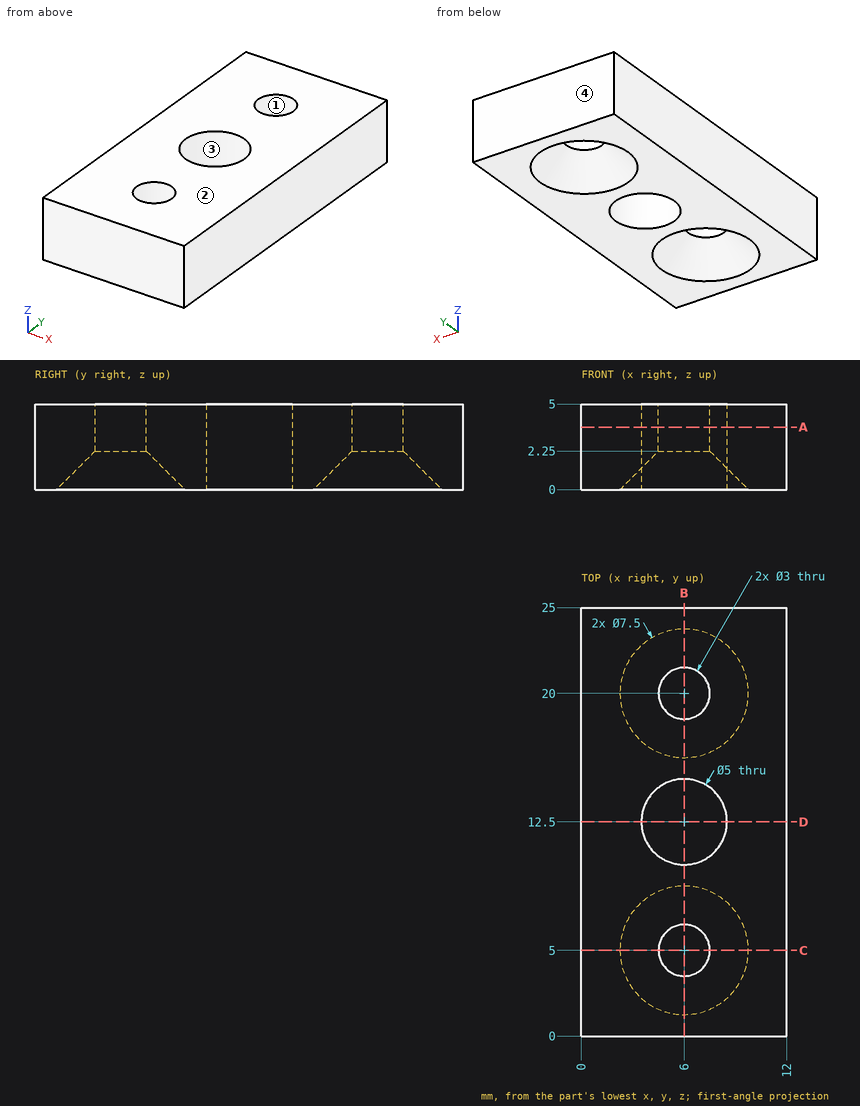
The figure shows three views and two pictorial views of one solid part (mm, origin at its lowest corner). Answer the questions. Round coordinates to 2 decimals unless told otherwise and drop trailing zeros. Write each loop counter-clockwise with the first axis right and the second up, starting at its lowest first coordinate (ties: lowest second). Pieces come first, ordered by that corner, then holes. Notation, with made-up numbers: (39.25, 22) -> (55.25, 22) arc R22 ccw to (55.25, 53) -> close; hole circle Ø4 at (-27.75, -29.75). An arc over 180 degrees is marked (long way). Answer as a JSON object with one key per item and string values. Group by question number.
Q1. Straight lines are drawn through the part: line 1 along Y through (x, z) = (6, 3.2); line 2 along X through (y, z) = (20, 3.85); line 3 along Y through (x, z) = (6.5, 4.35). For each, find the intervals that lie inside material, in ascending order.
Q2. Section B-B (x = 6) is taken. Write down the section's boundary in (y, z), plus the area to 3 significant figures.
Q3. Section A-A (z = 3.65) is taken. Write down the section's boundary in (x, y), plus the area to 3 significant figures.
Q4. Each of these flat-tipped pins is pushed along its axis until it touches: pin 1 Ø3.5 at (x, y) = (6, 20) entering from -Z; pin 2 Ø1.8 at (x, y) = (6, 5) entering from -Z (3 decimals). Where does it stop, or does it pass through?
Q5. Determine the mould class of the marked faces 1, 2, 3 and 4 for opening direction Y: pulls with the +Y half, pulls with the -Y half, needs draft (parallel to the pull), parting line crosses it, or undercut.
Q6. Section C-C (y = 5) is taken. Write down the section's boundary in (x, z).
Q7. Section D-D (y = 12.5) is taken. Write down the section's boundary in (x, z).
Check values:
{
 "1": {"line 1": "0 to 3.5, 6.5 to 10, 15 to 18.5, 21.5 to 25", "line 2": "0 to 4.5, 7.5 to 12", "line 3": "0 to 3.59, 6.41 to 10.05, 14.95 to 18.59, 21.41 to 25"},
 "2": {"outline": "(0, 0) -> (1.25, 0) -> (3.5, 2.25) -> (3.5, 5) -> (0, 5) -> close; (6.5, 2.25) -> (8.75, 0) -> (10, 0) -> (10, 5) -> (6.5, 5) -> close; (15, 0) -> (16.25, 0) -> (18.5, 2.25) -> (18.5, 5) -> (15, 5) -> close; (21.5, 2.25) -> (23.75, 0) -> (25, 0) -> (25, 5) -> (21.5, 5) -> close", "area": "59.9 mm^2"},
 "3": {"outline": "(0, 0) -> (12, 0) -> (12, 25) -> (0, 25) -> close; hole circle Ø5 at (6, 12.5); hole circle Ø3 at (6, 5); hole circle Ø3 at (6, 20)", "area": "266 mm^2"},
 "4": {"pin 1": "z = 2", "pin 2": "through"},
 "5": {"face 1": "undercut", "face 2": "needs draft", "face 3": "undercut", "face 4": "pulls with the +Y half"},
 "6": {"outline": "(0, 0) -> (2.25, 0) -> (4.5, 2.25) -> (4.5, 5) -> (0, 5) -> close; (7.5, 2.25) -> (9.75, 0) -> (12, 0) -> (12, 5) -> (7.5, 5) -> close"},
 "7": {"outline": "(0, 0) -> (3.5, 0) -> (3.5, 5) -> (0, 5) -> close; (8.5, 0) -> (12, 0) -> (12, 5) -> (8.5, 5) -> close"}
}
